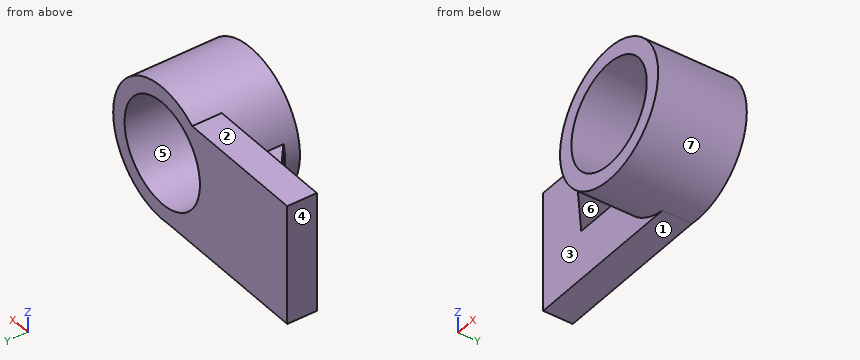
```python
from build123d import *

# Parameters (mm, degrees)
F0_R     = 22.27847408
F1_DEPTH = 38.1
F2_DEPTH = 12.7
F4_DEPTH = 19.05
F6_DEPTH = 25.4


with BuildPart() as f1:
    # F0 (on Front) → F1 (new body)
    with BuildSketch(Plane.XZ):
        with BuildLine():
            ThreePointArc((-3.4225089728, -28.7867356092), (19.2506230187, -21.674944708), (28.9894759301, 0))
            ThreePointArc((28.9894759301, 0), (12.795496455, 26.012785033), (-17.6940161623, 22.9632642878))
            ThreePointArc((-17.6940161623, 22.9632642878), (-27.9462435898, -7.7069568522), (-3.4225089728, -28.7867356092))
        make_face()
        Circle(F0_R, mode=Mode.SUBTRACT)
    extrude(amount=F1_DEPTH)

    # F0 (on Front) → F2 (join)
    with BuildSketch(Plane.XZ):
        with BuildLine():
            ThreePointArc((-3.4225089728, -28.7867356092), (-27.9462435898, -7.7069568522), (-17.6940161623, 22.9632642878))
            Line((-17.6940161623, 22.9632642878), (-73.8979172606, 22.9632642878))
            Line((-73.8979172606, 22.9632642878), (-73.8979172606, -28.7867356092))
            Line((-73.8979172606, -28.7867356092), (-3.4225089728, -28.7867356092))
        make_face()
    extrude(amount=F2_DEPTH)

    # F3 (on face) → F4 (join)
    with BuildSketch(Plane.XZ.offset(12.7)):
        with BuildLine():
            ThreePointArc((-27.9098332278, -7.8377882019), (-28.9873761892, -0.3489073921), (-28.0903995533, 7.1637397799))
            Line((-28.0903995533, 7.1637397799), (-51.3939457674, 7.1637397799))
            Line((-51.3939457674, 7.1637397799), (-51.3939457674, -7.8377882019))
            Line((-51.3939457674, -7.8377882019), (-27.9098332278, -7.8377882019))
        make_face()
    extrude(amount=F4_DEPTH)

    # F5 (on face) → F6 (cut)
    with BuildSketch(Plane(origin=(0, 0, -7.8377882019), x_dir=(1, 0, 0), z_dir=(0, 0, -1))):
        Polygon((-51.3939457674, 31.75), (-51.3939457674, 12.7), (-27.9098332278, 31.75), align=None)
    extrude(amount=-F6_DEPTH, mode=Mode.SUBTRACT)


solid = f1.part
```
Can you work these out from the model? Positions are in its coordinate system, mm. Face numbers are marked on the shaded views. A direction names the side the tool comes from. Coordinates: 2 decimals unless noted, no trailing zeros. Loops run counter-clockwise (first coordinate to the right, second up) from the corner with the lowest first, then second, coordinate; pieces in that order, holes last. Notation, with made-up numbers: (79.5, -29) - (131.5, -29) arc R29 ccw to (131.5, -4) - close; hole circle Ø3 at (45.25, 4). An arc over 180 degrees is marked (long way). Use a Markdown table: item, result.
Item 1: If I drill on probe 1 along Z at (x, y) = (0, -12.5); probe 2 along X at (y, z) = (-17, -13.5); probe 3 along X at (y, z) = (-5, 3), over which ranges is the centre line in solid material (lowest first)? Write a range as from..to.
Numbers:
| item | result |
|---|---|
| probe 1 | z = -28.99..-22.28, 22.28..28.99 |
| probe 2 | x = -25.65..-17.72, 17.72..25.65 |
| probe 3 | x = -73.9..-22.08, 22.08..28.83 |
Item 2: Will these pins go through, and if not, where does the flat tip stop? pin 1 (1 mm diameter, centred on x = -51, z = -9.5, fed in from -Y); pin 2 (14 mm diameter, centred on x = -48, y = -4.5, fed in from +Z); pin 3 (6.5 mm diameter, centred on x = -24, y = -8.5, fed in from -Z); pin 4 (0.9 mm diameter, centred on x = -28.5, z = -4, fed in from +Y).
Numbers:
| item | result |
|---|---|
| pin 1 | stops at y = -12.7 |
| pin 2 | stops at z = 22.96 |
| pin 3 | stops at z = -28.79 |
| pin 4 | stops at y = 0 |
Item 3: I want a section at C-C on y = -11. Please give me the cut outline in (x, z), and give its area (3 significant figures).
Numbers:
| item | result |
|---|---|
| outline | (-73.9, -28.79) - (-3.42, -28.79) arc R28.99 ccw (long way) to (-17.69, 22.96) - (-73.9, 22.96) - close; hole circle Ø44.56 at (0, 0) |
| area | 3,660 mm2 |
Item 4: We'd pull the mould along X, two halves only. Please class the marked faces 4, 5, 6 and 7: released by +X, released by -X, zero draft, split by the parting line, or undercut.
Numbers:
| item | result |
|---|---|
| face 4 | released by -X |
| face 5 | undercut |
| face 6 | zero draft |
| face 7 | split by the parting line |
Item 5: For the marked faces 1, 2 and 3, which set-ups out of +Z, -Z, +X, -X, +Y, -Y let a thin tool reach every point of the face, with its end or its side?
Numbers:
| item | result |
|---|---|
| face 1 | -Z, -X, +Y, -Y |
| face 2 | +Z, -X, +Y, -Y |
| face 3 | -X, -Y |
Item 6: I want a section at A-A on x = 0. Please give me the cut outline in (y, z), and give its area (3 significant figures).
Numbers:
| item | result |
|---|---|
| outline | (-38.1, -28.99) - (0, -28.99) - (0, -22.28) - (-38.1, -22.28) - close; (-38.1, 22.28) - (0, 22.28) - (0, 28.99) - (-38.1, 28.99) - close |
| area | 511 mm2 |
Item 7: I want a section at D-D on x = -12.5. Please give me the cut outline in (y, z).
Numbers:
| item | result |
|---|---|
| outline | (-38.1, -26.16) - (-12.7, -26.16) - (-12.7, -28.79) - (0, -28.79) - (0, -18.44) - (-38.1, -18.44) - close; (-38.1, 18.44) - (0, 18.44) - (0, 26.16) - (-38.1, 26.16) - close |
Item 8: I want a section at B-B on z = 0. Please give me the cut outline in (x, y), and give its area (3 significant figures).
Numbers:
| item | result |
|---|---|
| outline | (-73.9, -12.7) - (-51.39, -12.7) - (-27.91, -31.75) - (-28.99, -31.75) - (-28.99, -38.1) - (-22.28, -38.1) - (-22.28, 0) - (-73.9, 0) - close; (22.28, -38.1) - (28.99, -38.1) - (28.99, 0) - (22.28, 0) - close |
| area | 1,280 mm2 |
